For this review, take the finished solid that the model builds, in its own axes (mm). Face numbers are marked on the shaded views. A direction names the side the tool comes from. Coordinates: 2 decimals unless noted, no trailing zeros. Write each loop counter-clockwise with the first axis right and the second up, starting at its lowest first coordinate (ties: lowest second). Pieces come first, ordered by that corner, then holes. Notation, with made-up numbers: (-34, 63.5) -> (7, 63.5) arc R15 cw to (7, 77.5) -> close; hole circle Ø6 at (9, 27.5). An arc over 180 degrees is marked (long way). Put each result on its own line as item: value. Start each with the question number.
Item 1: Consider section D-D on z = -4. Give the boundary of the cut face in (x, y).
Item 2: For the marked faces 1 and 2, list the 3-axis set-ups (+Z, -Z, +X, -X, +Y, -Y) from which the entire face can be reached by the end or side of a thin tool; tool diameter is ignored.
Item 3: Consider section A-A on y = 22.8. Give the boundary of the cut face in (x, z), and give its area (3 significant figures).
Item 4: To check wall thickness, follow L1, parallel to Z at x = 23.85, y = 22.8; L2, parallel to X at y = 11, z = 11.5; L3, parallel to Y at x = 13.5, z = 13. State the ranges of each line that lie inside material, in increasing order.
Item 5: Consider section B-B on y = 14.5. Give the boundary of the cut face in (x, z).
Item 6: The part is to be moulded in two halves that separate along X. For the marked faces 3, 4, 5 and 6, say which applies: +X half, -X half, draft (parallel to the pull), parting line (faces both ways), or undercut.
Item 7: Insertion check: P1, Ø13.5, axis at x = -5.5, z = -9, coming from the +Y side. The pin has a flat end and moves straight along its axis. Give the tip position at first contact, or say it passes through.
Item 8: Consider section C-C on z = -10.99. Give the boundary of the cut face in (x, y), and give its area (3 significant figures).
```python
from build123d import *

# Parameters (mm, degrees)
BOSS_EXTRUDE1_DEPTH = 28.5
SKETCH2_R           = 4
CUT_EXTRUDE1_DEPTH  = 68.6546226


with BuildPart() as part:
    # Sketch1 → Boss-Extrude1 (new, symmetric)
    with BuildSketch(Plane.XY):
        Polygon((-26, 0), (26, 0), (26, 32.571428571), (22.533333333, 32.571428571), (22.533333333, 3.466666667), (-22.533333333, 3.466666667), (-22.533333333, 32.571428571), (-26, 32.571428571), align=None)
    extrude(amount=BOSS_EXTRUDE1_DEPTH, both=True)

    # Sketch2 → Cut-Extrude1 (cut, through all)
    with BuildSketch(Plane(origin=(26, 0, 0), x_dir=(0, 0, -1), z_dir=(1, 0, 0))):
        with Locations(Location((-10.99, 22.8, 0), (0, 0, 90))):
            Circle(SKETCH2_R)
        with Locations(Location((10.99, 22.8, 0), (0, 0, 270))):
            Circle(SKETCH2_R)
    extrude(amount=-CUT_EXTRUDE1_DEPTH, mode=Mode.SUBTRACT)


solid = part.part
```
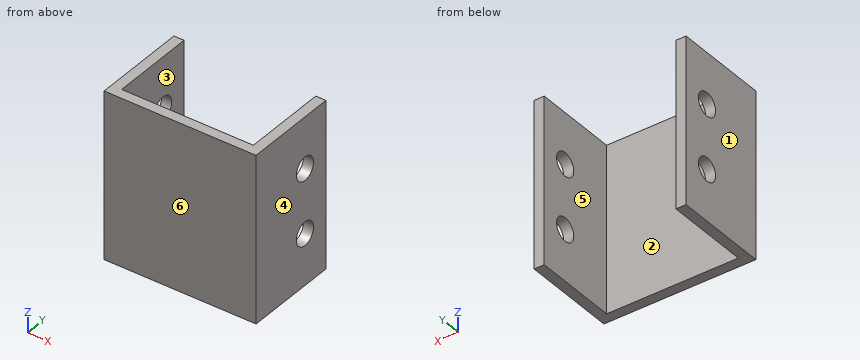
Return value:
1. outline: (-26, 0) -> (26, 0) -> (26, 32.57) -> (22.53, 32.57) -> (22.53, 3.47) -> (-22.53, 3.47) -> (-22.53, 32.57) -> (-26, 32.57) -> close
2. face 1: +Z, -Z, -X, +Y, -Y
2. face 2: +Z, -Z, +Y
3. outline: (-26, -28.5) -> (-22.53, -28.5) -> (-22.53, -14.99) -> (-26, -14.99) -> close; (-26, -6.99) -> (-22.53, -6.99) -> (-22.53, 6.99) -> (-26, 6.99) -> close; (-26, 14.99) -> (-22.53, 14.99) -> (-22.53, 28.5) -> (-26, 28.5) -> close; (22.53, -28.5) -> (26, -28.5) -> (26, -14.99) -> (22.53, -14.99) -> close; (22.53, -6.99) -> (26, -6.99) -> (26, 6.99) -> (22.53, 6.99) -> close; (22.53, 14.99) -> (26, 14.99) -> (26, 28.5) -> (22.53, 28.5) -> close
3. area: 284 mm^2
4. L1: -28.5 to -14.99, -6.99 to 6.99, 14.99 to 28.5
4. L2: -26 to -22.53, 22.53 to 26
4. L3: 0 to 3.47
5. outline: (-26, -28.5) -> (-22.53, -28.5) -> (-22.53, 28.5) -> (-26, 28.5) -> close; (22.53, -28.5) -> (26, -28.5) -> (26, 28.5) -> (22.53, 28.5) -> close
6. face 3: undercut
6. face 4: +X half
6. face 5: undercut
6. face 6: draft
7. P1: y = 3.47
8. outline: (-26, 0) -> (26, 0) -> (26, 18.8) -> (22.53, 18.8) -> (22.53, 3.47) -> (-22.53, 3.47) -> (-22.53, 18.8) -> (-26, 18.8) -> close; (-26, 26.8) -> (-22.53, 26.8) -> (-22.53, 32.57) -> (-26, 32.57) -> close; (22.53, 26.8) -> (26, 26.8) -> (26, 32.57) -> (22.53, 32.57) -> close
8. area: 327 mm^2
